from build123d import *

# Parameters (mm, degrees)
F0_W     = 210
F0_H     = 210
F1_DEPTH = 0.8
F2_W     = 210
F2_H     = 210
F2_W_2   = 207.12
F2_H_2   = 207.12
F3_DEPTH = 2
F4_W     = 15
F4_H     = 1.44
F4_W_2   = 23.556538
F5_DEPTH = 2
F6_W     = 71.4
F6_H     = 21
F7_DEPTH = 0.8


with BuildPart() as f1:
    # F0 (on Top) → F1 (new body)
    with BuildSketch(Plane.XY):
        with Locations((105, 105)):
            Rectangle(F0_W, F0_H)
    extrude(amount=F1_DEPTH)

    # F2 (on face) → F3 (join)
    with BuildSketch(Plane.XY.offset(0.8)):
        with Locations((105, 105)):
            Rectangle(F2_W, F2_H)
        with Locations((105, 105)):
            Rectangle(F2_W_2, F2_H_2, mode=Mode.SUBTRACT)
    extrude(amount=F3_DEPTH)

    # F4 (on face) → F5 (join, through all)
    with BuildSketch(Plane.XY.offset(0.8)):
        Polygon((74.28, 156.72), (74.28, 208.56), (72.84, 208.56), (72.84, 158.16), (35.766923, 158.16), (35.766923, 132.3), (1.44, 132.3), (1.44, 130.86), (35.766923, 130.86), (60.966923, 130.86), (60.966923, 111.96), (45.966923, 111.96), (45.966923, 110.52), (62.406923, 110.52), (62.406923, 130.86), (62.406923, 132.3), (37.206923, 132.3), (37.206923, 156.72), align=None)
        with Locations((8.94, 111.24)):
            Rectangle(F4_W, F4_H)
        Polygon((208.56, 150.581538), (208.56, 152.021538), (100.56, 152.021538), (100.56, 183.56), (99.12, 183.56), (99.12, 145.581538), (100.56, 145.581538), (100.56, 150.581538), (136.446923, 150.581538), (136.446923, 102.941538), (160.003462, 102.941538), (160.003462, 104.381538), (137.886923, 104.381538), (137.886923, 150.581538), align=None)
        with Locations((196.781731, 103.661538)):
            Rectangle(F4_W_2, F4_H)
        Polygon((91.44, 1.44), (92.88, 1.44), (92.88, 118.555385), (102.88, 118.555385), (102.88, 119.995385), (86.44, 119.995385), (86.44, 118.555385), (91.44, 118.555385), align=None)
    extrude(amount=F5_DEPTH)

    # F6 (on face) → F7 (join)
    with BuildSketch(Plane.XY.offset(0.8)):
        with Locations((37.14, 198.06)):
            Rectangle(F6_W, F6_H)
    extrude(amount=F7_DEPTH)


solid = f1.part
The listing builds one solid part. Answer for the finished solid, in the listing's coordinates (mm). Coordinates: 2 decimals unless noted, no trailing zeros. Loops run counter-clockwise (first coordinate to the right, second up) from the corner with the lowest first, then second, coordinate; pieces in that order, holes last. Notation, with made-up numbers: (42.25, 55) -> (98.25, 55) arc R15 ccw to (98.25, 61) -> close; hole circle Ø6 at (88.25, 77.25). An arc over 180 degrees is marked (long way). Write item = value, one per line. Start each with the question number.
1) A cutting plane is placed at A-A (x = 58.5). Give the vertices of the cut face in (y, z), then the cut area to 3 significant figures.
2) A cutting plane is placed at B-B (y = 25.5). Give the vertices of the cut face in (x, z).
3) A cutting plane is placed at C-C (z = 2.1). Count the separate pieces of the cut face and the enclosed holes in it, then the cut area to 3 significant figures.
4) The mould has two halves that part along X. Classify faces 1 (the face through (104, 106, 0)), 2 (the face through (37, 198, 1.6)): released by +X, released by -X, zero draft, split by the parting line, or undercut.
5) Given pin 1 Ø4 at (x, y) = (179, 103.5) entering from +Z, flat-ended and moving along its own axis, determine where the tip first touches the part or whether it passes through.
6) Straight lines are drawn through the part: line 1 (Y direction, x = 166, z = 2); line 2 (Y direction, x = 151, z = 1.65); line 3 (X direction, y = 69, z = 0.95). For each, find the intervals that lie inside material, in ascending order. Write a range as from..to.
7) A cutting plane is placed at D-D (x = 182.5). Give the vertices of the cut face in (y, z).
Responses:
q1.outline = (0, 0) -> (210, 0) -> (210, 2.8) -> (208.56, 2.8) -> (208.56, 1.6) -> (187.56, 1.6) -> (187.56, 0.8) -> (158.16, 0.8) -> (158.16, 2.8) -> (156.72, 2.8) -> (156.72, 0.8) -> (132.3, 0.8) -> (132.3, 2.8) -> (130.86, 2.8) -> (130.86, 0.8) -> (111.96, 0.8) -> (111.96, 2.8) -> (110.52, 2.8) -> (110.52, 0.8) -> (1.44, 0.8) -> (1.44, 2.8) -> (0, 2.8) -> close
q1.area = 199 mm²
q2.outline = (0, 0) -> (210, 0) -> (210, 2.8) -> (208.56, 2.8) -> (208.56, 0.8) -> (92.88, 0.8) -> (92.88, 2.8) -> (91.44, 2.8) -> (91.44, 0.8) -> (1.44, 0.8) -> (1.44, 2.8) -> (0, 2.8) -> close
q3.separate_pieces = 1
q3.enclosed_holes = 2
q3.area = 2,060 mm²
q4.face_1 = zero draft
q4.face_2 = undercut
q5.pin_1 = 0.8
q6.line_1 = 0..1.44, 150.58..152.02, 208.56..210
q6.line_2 = 0..1.44, 102.94..104.38, 150.58..152.02, 208.56..210
q6.line_3 = 0..1.44, 91.44..92.88, 208.56..210
q7.outline = (0, 0) -> (210, 0) -> (210, 2.8) -> (208.56, 2.8) -> (208.56, 0.8) -> (152.02, 0.8) -> (152.02, 2.8) -> (150.58, 2.8) -> (150.58, 0.8) -> (1.44, 0.8) -> (1.44, 2.8) -> (0, 2.8) -> close
